from build123d import *

# Parameters (mm, degrees)
SKETCH1_W           = 63.5
SKETCH1_H           = 25.4
BOSS_EXTRUDE1_DEPTH = 3.175
SKETCH2_W           = 63.5
SKETCH2_H           = 3.175
BOSS_EXTRUDE2_DEPTH = 22.225
SKETCH3_R           = 3.175
CUT_EXTRUDE1_DEPTH  = 3.175
SKETCH4_R           = 3.175
CUT_EXTRUDE2_DEPTH  = 3.175


with BuildPart() as part:
    # Sketch1 → Boss-Extrude1 (new body)
    with BuildSketch(Plane(origin=(0, 0, 0), x_dir=(1, 0, 0), z_dir=(0, 1, 0))):
        Rectangle(SKETCH1_W, SKETCH1_H)
    extrude(amount=BOSS_EXTRUDE1_DEPTH)

    # Sketch2 → Boss-Extrude2 (add)
    with BuildSketch(Plane(origin=(0, 3.175, 0), x_dir=(1, 0, 0), z_dir=(0, 1, 0))):
        with Locations((0, -11.1125)):
            Rectangle(SKETCH2_W, SKETCH2_H)
    extrude(amount=BOSS_EXTRUDE2_DEPTH)

    # Sketch3 → Cut-Extrude1 (cut)
    with BuildSketch(Plane(origin=(0, 0, 9.525), x_dir=(-1, 0, 0), z_dir=(0, 0, -1))):
        with Locations((6.35, 12.7)):
            Circle(SKETCH3_R)
        with Locations((-6.35, 12.7)):
            Circle(SKETCH3_R)
    extrude(amount=-CUT_EXTRUDE1_DEPTH, mode=Mode.SUBTRACT)

    # Sketch4 → Cut-Extrude2 (cut)
    with BuildSketch(Plane(origin=(0, 3.175, 0), x_dir=(1, 0, 0), z_dir=(0, 1, 0))):
        with Locations(Location((-19.05, 0, 0), (0, 0, 270))):
            Circle(SKETCH4_R)
        with Locations(Location((19.05, 3.175, 0), (0, 0, 270))):
            Circle(SKETCH4_R)
    extrude(amount=-CUT_EXTRUDE2_DEPTH, mode=Mode.SUBTRACT)


solid = part.part
Check sheet for the modelled part. Datum: model origin and axes. Units: mm. A direction names the side the tool comes from. Give positions to 0.01 mm unless a question says otherwise; leave off trailing zeros. Order: outer loops, then holes, each group sorted by start corner. A loop starts at its lowest first (then second) coordinate and runs counter-clockwise, first axis right, second up. Notation, with made-up numbers: M 84,-6 L 112,-6 A10 cw 112,0 Z; hole C 70,2 d4. An arc over 180 degrees is marked long. Answer as CSV lines item,"result". Start each with the question number.
Item 1: Tool access check on faces 4 (the face through (0, 14, 9.525)), 5 (the face through (4.885, 9.883, 11.09)). Record the directions out of +Z, -Z, +X, -X, +Y, -Y that give a thin tool (end or side, any length) a straight path to the whole face; none if there is none.
Item 2: Cross-section at B-B on y = 12.7. Enter the section's corners in (x, z) (3 decimals).
Item 3: Cross-section at A-A on x = -6.35. Enter the section's corners in (y, z) (3 decimals), plus the area to 3 significant figures.
Item 4: Cross-section at C-C on z = -5. Enter the section's corners in (x, y) (3 decimals), plus the area to 3 significant figures.
Item 5: Gauge pin test, flat ends, axial feed: P1, Ø10, axis at x = 6.35, y = 12.7, coming from the -Z side (3 decimals); P2, Ø3, axis at x = 7.5, z = 6.5, coming from the +Y side (3 decimals). Record the tip position at first contact, or that the pin passes through.
Item 6: Thickness scan on line 1 (X direction, y = 13, z = 10); line 2 (Y direction, x = -6.35, z = 10.8) (3 decimals); line 3 (Z direction, x = -5.5, y = 22.75) (3 decimals). Record the ranges inside material, lowest first. Write a range as [from, to].
Item 7: Cross-section at D-D on x = -17. Enter the section's corners in (y, z) (3 decimals).
Item 8: Mould release check, pull along X, two halves, no side actions. Record for faces 1 (the face through (-31.75, 7, 10)), 2 (the face through (0, 3.175, -2)), 3 (the face through (-18.1, 1.61, 3.03)): +X half, -X half, draft (parallel to the pull), parting line (faces both ways), or undercut.
Established:
1,face 4,"-Z, +X, -X, +Y"
1,face 5,"+Z, -Z"
2,outline,"M -31.75,9.525 L -9.525,9.525 L -9.525,12.7 L -31.75,12.7 Z; M -3.175,9.525 L 3.175,9.525 L 3.175,12.7 L -3.175,12.7 Z; M 9.525,9.525 L 31.75,9.525 L 31.75,12.7 L 9.525,12.7 Z"
3,outline,"M 0,-12.7 L 3.175,-12.7 L 3.175,9.525 L 9.525,9.525 L 9.525,12.7 L 0,12.7 Z; M 15.875,9.525 L 25.4,9.525 L 25.4,12.7 L 15.875,12.7 Z"
3,area,"131 mm^2"
4,outline,"M -31.75,0 L 16.452,0 L 16.452,3.175 L -31.75,3.175 Z; M 21.648,0 L 31.75,0 L 31.75,3.175 L 21.648,3.175 Z"
4,area,"185 mm^2"
5,P1,"stops at z = 9.525"
5,P2,"stops at y = 3.175"
6,line 1,"x = [-31.75, -9.51], [-3.19, 3.19], [9.51, 31.75]"
6,line 2,"y = [0, 9.525], [15.875, 25.4]"
6,line 3,"z = [9.525, 12.7]"
7,outline,"M 0,-12.7 L 3.175,-12.7 L 3.175,-2.424 L 0,-2.424 Z; M 0,2.424 L 3.175,2.424 L 3.175,9.525 L 25.4,9.525 L 25.4,12.7 L 0,12.7 Z"
8,face 1,"-X half"
8,face 2,"draft"
8,face 3,"undercut"
